Autodesk Fusion 360 part; units mm, degrees
sketch "Sketch1" plane through (0, 0, 0) normal (0, 1, 0) x (1, 0, 0)
  line L0 (0, 0) -> (30, 0)
  line L1 (30, 0) -> (30, -30)
  line L2 (30, -30) -> (0, -30)
  line L3 (0, -30) -> (0, 0)
  line L4 (3.2, -3.2) -> (26.8, -3.2)
  line L5 (26.8, -3.2) -> (26.8, -26.8)
  line L6 (26.8, -26.8) -> (3.2, -26.8)
  line L7 (3.2, -26.8) -> (3.2, -3.2)
  dimension "d1" = 30
  dimension "d2" = 30
  dimension "d3" = 3.2
  dimension "d4" = 3.2
  dimension "d5" = 3.2
  dimension "d6" = 3.2
extrude "Extrude1" add sketch "Sketch1" along normal blind 50 makes body 1
sketch "Sketch2" plane through (0, 0, 30) normal (0, 0, 1) x (1, 0, 0)
  line L0 (0, 0) -> (30, 0)
  line L1 (30, 0) -> (30, 50)
  line L2 (30, 50) -> (0, 50)
  line L3 (0, 50) -> (0, 0)
  line L4 (10, 3.2) -> (20, 3.2)
  line L5 (20, 3.2) -> (20, 21.2)
  line L6 (20, 21.2) -> (10, 21.2)
  line L7 (10, 21.2) -> (10, 3.2)
  line L8 (5, 44) -> (12.5, 44)
  line L9 (12.5, 44) -> (12.5, 36.5)
  line L10 (12.5, 36.5) -> (5, 36.5)
  line L11 (5, 36.5) -> (5, 44)
  line L12 (17.5, 44) -> (25, 44)
  line L13 (25, 44) -> (25, 36.5)
  line L14 (25, 36.5) -> (17.5, 36.5)
  line L15 (17.5, 36.5) -> (17.5, 44)
  line L16 (0, 50) -> (-2.5, 50)
  line L17 (30, 50) -> (32.5, 50)
  line L18 (-2.5, 50) -> (15, 70)
  line L19 (15, 70) -> (32.5, 50)
  dimension "d9" = 18
  dimension "d10" = 10
  dimension "d11" = 10
  dimension "d12" = 3.2
  dimension "d13" = 7.5
  dimension "d14" = 7.5
  dimension "d15" = 5
  dimension "d16" = 6
  dimension "d17" = 7.5
  dimension "d18" = 7.5
  dimension "d19" = 5
  dimension "d20" = 6
  dimension "d51" = 2.5
  dimension "d52" = 2.5
  dimension "d53" = 17.5
  dimension "d54" = 20
extrude "Extrude2" cut sketch "Sketch2" against normal blind 3.2 contours L4 L5 L6 L7 bodies 1
extrude "Extrude3" add sketch "Sketch1" along normal blind 3.2 contours L4 L5 L6 L7 bodies 1
extrude "Extrude4" cut sketch "Sketch2" against normal blind 3.2 contours L8 L9 L10 L11 | L12 L13 L14 L15 bodies 1
sketch "Sketch3" plane through (30, 0, 0) normal (1, 0, 0) x (0, 0, -1)
  line L0 (-30, 0) -> (0, 0)
  line L1 (0, 0) -> (0, 50)
  line L2 (0, 50) -> (-30, 50)
  line L3 (-30, 50) -> (-30, 0)
  line L4 (-25, 21.2) -> (-17.5, 21.2)
  line L5 (-17.5, 21.2) -> (-17.5, 13.7)
  line L6 (-17.5, 13.7) -> (-25, 13.7)
  line L7 (-25, 13.7) -> (-25, 21.2)
  line L8 (-12.5, 21.2) -> (-5, 21.2)
  line L9 (-5, 21.2) -> (-5, 13.7)
  line L10 (-5, 13.7) -> (-12.5, 13.7)
  line L11 (-12.5, 13.7) -> (-12.5, 21.2)
  line L12 (-30, 3.2) -> (-30, 21.2)
  line L13 (0, 0) -> (-30, 0)
  line L14 (-18.75, 44) -> (-11.25, 44)
  line L15 (-11.25, 44) -> (-11.25, 36.5)
  line L16 (-11.25, 36.5) -> (-18.75, 36.5)
  line L17 (-18.75, 36.5) -> (-18.75, 44)
  dimension "d27" = 7.5
  dimension "d28" = 7.5
  dimension "d29" = 5
  dimension "d30" = 5
  dimension "d31" = 7.5
  dimension "d32" = 7.5
  dimension "d33" = 13.7
  dimension "d34" = 13.7
  dimension "d35" = 6
  dimension "d36" = 7.5
  dimension "d37" = 7.5
  dimension "d38" = 11.25
extrude "Extrude5" cut sketch "Sketch3" against normal blind 30 contours L14 L15 L16 L17 bodies 1
extrude "Extrude6" cut sketch "Sketch3" against normal blind 30 contours L4 L5 L6 L7 | L8 L9 L10 L11 bodies 1
sketch "Sketch4" plane through (0, 50, 0) normal (0, 1, 0) x (-1, 0, 0)
  line L0 (-26.8, 26.8) -> (-3.2, 26.8)
  line L1 (-3.2, 26.8) -> (-3.2, 3.2)
  line L2 (-3.2, 3.2) -> (-26.8, 3.2)
  line L3 (-26.8, 3.2) -> (-26.8, 26.8)
  line L4 (0, 30) -> (-30, 30)
  line L5 (-30, 30) -> (-30, 0)
  line L6 (-30, 0) -> (0, 0)
  line L7 (0, 0) -> (0, 30)
  line L8 (2.5, -2.5) -> (-32.5, -2.5)
  line L9 (-32.5, -2.5) -> (-32.5, 32.5)
  line L10 (-32.5, 32.5) -> (2.5, 32.5)
  line L11 (2.5, 32.5) -> (2.5, -2.5)
  line L12 (0, 30) -> (0, 0)
  line L13 (0, 0) -> (-30, 0)
  line L14 (-30, 0) -> (-30, 30)
  line L15 (-30, 30) -> (0, 30)
  line L16 (-18.3, 8.2) -> (-25.8, 8.2)
  line L17 (-25.8, 8.2) -> (-25.8, 15.7)
  line L18 (-25.8, 15.7) -> (-18.3, 15.7)
  line L19 (-18.3, 15.7) -> (-18.3, 8.2)
  line L20 (-26.8, 26.8) -> (-3.2, 26.8)
  line L21 (-26.8, 3.2) -> (-26.8, 26.8)
  line L22 (-3.2, 3.2) -> (-26.8, 3.2)
  dimension "d43" = 2.5
  dimension "d44" = 2.5
  dimension "d45" = 2.5
  dimension "d46" = 2.5
  dimension "d47" = 7.5
  dimension "d48" = 7.5
  dimension "d59" = 1
  dimension "d60" = 5
extrude "Extrude7" add sketch "Sketch2" along normal blind 2.5 separate body contours L2 L16 L17 L18 L19 makes body 2
extrude "Extrude8" add sketch "Sketch2" against normal blind 32.5 contours L2 L16 L17 L18 L19 bodies 1 2
extrude "Extrude9" add sketch "Sketch4" along normal blind 21.5 contours L16 L17 L18 L19 bodies 1
Model file for the job. Use its own axes, mm. A direction names the side the tool comes from. Give positions to 0.01 mm unless a question says otherwise; leave off trailing zeros. Order: outer loops, then holes, each group sorted by start corner. A loop starts at its lowest first (then second) coordinate and runs counter-clockwise, first axis right, second up.
1) 3-axis set-ups, long thin cutter, end or side, ignore diameter. For faces 4 (the flat face through (2, 40, 11.25)), 5 (the flat face through (21, 44, 28)), 6 (the flat face through (15, 50, 15)): which of +Z, -Z, +X, -X, +Y, -Y reach the whole face in a straight line?
2) Pin check, flat tips, straight feed: pin 1 (3.5 mm diameter, centred on x = 2, y = 16, fed in from -Z); pin 2 (2.5 mm diameter, centred on x = 1.5, z = 20, fed in from +Y); pin 3 (2.5 mm diameter, centred on x = 1.5, y = 41.5, fed in from +Z). Stop position of each tip, or through.
3) Saw through at C-C, the plane z = 26. Write the cut outline in (x, y).
4) Saw through at D-D, the plane y = 6.5. Write the cut outline in (x, z).
5) Saw through at A-A, the plane z = 7.5. Write the cut outline in (x, y).
6) Saw through at B-B, the plane y = 19. Write the cut outline in (x, z).
7) Mould opens along Y. For faces 1 (the flat face through (12.5, 40, 28)), 2 (the flat face through (15, 25, 30)), 3 (the flat face through (6.13, 59.86, 14.76)) say: +Y half, -Y half, draft (parallel to the pull), parting line (faces both ways), or undercut.
8) Wall check: probe 1 along X at (y, z) = (37, 20.5); probe 2 along Y at (x, z) = (1, 12). Give the ranges that are in metal, low to high.
Computed:
1. face 4: +X, -X
1. face 5: +Z
1. face 6: none
2. pin 1: stops at z = 0
2. pin 2: stops at y = 56
2. pin 3: stops at z = 30
3. outline: (-2.5, 50) - (0, 50) - (0, 0) - (30, 0) - (30, 50) - (32.5, 50) - (15, 70) - close; hole (3.2, 3.2) - (26.8, 3.2) - (26.8, 50) - (3.2, 50) - close
4. outline: (0, 0) - (30, 0) - (30, 30) - (20, 30) - (20, 26.8) - (26.8, 26.8) - (26.8, 3.2) - (3.2, 3.2) - (3.2, 26.8) - (10, 26.8) - (10, 30) - (0, 30) - close
5. outline: (-2.5, 50) - (0, 50) - (0, 21.2) - (3.2, 21.2) - (3.2, 50) - (26.8, 50) - (26.8, 21.2) - (30, 21.2) - (30, 50) - (32.5, 50) - (15, 70) - close; (0, 0) - (30, 0) - (30, 13.7) - (26.8, 13.7) - (26.8, 3.2) - (3.2, 3.2) - (3.2, 13.7) - (0, 13.7) - close
6. outline: (0, 0) - (30, 0) - (30, 5) - (26.8, 5) - (26.8, 3.2) - (3.2, 3.2) - (3.2, 5) - (0, 5) - close; (0, 12.5) - (3.2, 12.5) - (3.2, 17.5) - (0, 17.5) - close; (0, 25) - (3.2, 25) - (3.2, 26.8) - (10, 26.8) - (10, 30) - (0, 30) - close; (20, 26.8) - (26.8, 26.8) - (26.8, 25) - (30, 25) - (30, 30) - (20, 30) - close; (26.8, 12.5) - (30, 12.5) - (30, 17.5) - (26.8, 17.5) - close
7. face 1: undercut
7. face 2: draft
7. face 3: +Y half
8. probe 1: x = 0 to 3.2, 26.8 to 30
8. probe 2: y = 0 to 13.7, 21.2 to 36.5, 44 to 54
